Read the model definition and answer for the solid it produces. Units are mm, in the model's axes. A direction names the side the tool comes from. Give positions to 0.01 mm unless a question says otherwise; leave off trailing zeros. Order: outer loops, then holes, each group sorted by start corner. A loop starts at its lowest first (then second) coordinate and runs counter-clockwise, first axis right, second up. Notation, with made-up numbers: (-38, 31.25) - (1, 31.25) arc R23 cw to (1, 69.25) - close; hole circle Ø6 at (-9.75, 46.5). An arc over 180 degrees is marked (long way). Return JSON: item names as keys, results as strings.
```python
from build123d import *

# Parameters (mm, degrees)
F1_DEPTH  = 38.1
F2_W      = 69.85
F2_H      = 69.85
F3_DEPTH  = 127
F5_DEPTH  = 76.2
F7_DEPTH  = 25.4
F8_W      = 3.175
F8_H      = 190.3737529909
F9_DEPTH  = 3.175
F10_W     = 4.2661567543
F10_H     = 3.175
F11_DEPTH = 76.2


with BuildPart() as f1:
    # F0 (on Right) → F1 (new body, symmetric)
    with BuildSketch(Plane.YZ):
        Polygon((-76.2, 38.1), (-101.6, -38.1), (101.6, -38.1), (76.2, 38.1), align=None)
    extrude(amount=F1_DEPTH, both=True)

    # F2 (on Front) → F3 (cut, symmetric)
    with BuildSketch(Plane.XZ):
        Rectangle(F2_W, F2_H)
    extrude(amount=F3_DEPTH, both=True, mode=Mode.SUBTRACT)

    # F4 (on face) → F5 (cut)
    with BuildSketch(Plane(origin=(-38.1, 0, 0), x_dir=(0, -1, 0), z_dir=(-1, 0, 0))):
        Polygon((-71.9035431621, 34.925), (-95.1868764954, -34.925), (-71.9035431621, -34.925), align=None)
        Polygon((-66.8235431621, 27.423295483), (-66.8235431621, -34.925), (-38.1337124981, -3.7508522585), align=None)
        Polygon((-2.54, 34.925), (-66.8235431621, 34.925), (-34.6817715811, 0), align=None)
        Polygon((-2.54, -34.925), (-2.54, 27.423295483), (-31.229830664, -3.7508522585), align=None)
        Polygon((-34.6817715811, -7.501704517), (-59.9196613281, -34.925), (-9.443881834, -34.925), align=None)
        Polygon((31.229830664, -3.7508522585), (2.54, 27.423295483), (2.54, -34.925), align=None)
        Polygon((66.8235431621, 34.925), (2.54, 34.925), (34.6817715811, 0), align=None)
        Polygon((66.8235431621, -34.925), (66.8235431621, 27.423295483), (38.1337124981, -3.7508522585), align=None)
        Polygon((34.6817715811, -7.501704517), (9.443881834, -34.925), (59.9196613281, -34.925), align=None)
        Polygon((95.1868764954, -34.925), (71.9035431621, 34.925), (71.9035431621, -34.925), align=None)
    extrude(amount=-F5_DEPTH, mode=Mode.SUBTRACT)

    # F6 (on face) → F7 (cut)
    with BuildSketch(Plane.XY.offset(38.1)):
        Polygon((-34.925, 73.025), (-34.925, -58.3073754949), (-3.5194319469, 7.3588122526), align=None)
        Polygon((-34.925, -73.025), (34.925, -73.025), (0, 0), align=None)
        Polygon((3.5194319469, 7.3588122526), (34.925, -58.3073754949), (34.925, 73.025), align=None)
        Polygon((0, 14.7176245051), (27.8861361062, 73.025), (-27.8861361062, 73.025), align=None)
    extrude(amount=-F7_DEPTH, mode=Mode.SUBTRACT)

    # F8 (on face) → F9 (join)
    with BuildSketch(Plane.XY.offset(-34.925)):
        with Locations((-36.5125, 0)):
            Rectangle(F8_W, F8_H)
        with Locations((36.5125, 0)):
            Rectangle(F8_W, F8_H)
    extrude(amount=F9_DEPTH)

    # F10 (on face) → F11 (join)
    with BuildSketch(Plane.YZ.offset(38.1)):
        with Locations((-99.4669216229, -36.5125)):
            Rectangle(F10_W, F10_H)
        with Locations((99.4669216229, -36.5125)):
            Rectangle(F10_W, F10_H)
    extrude(amount=-F11_DEPTH)


solid = f1.part
```
Q1. A cutting plane is placed at A-A (x = -25). Write down the section's boundary in (y, z) (3 decimals), and give its area (3 significant figures).
Values:
{"outline": "(-101.6, -38.1) - (101.6, -38.1) - (101.6, -34.925) - (-101.6, -34.925) - close; (-77.258, 34.925) - (-73.025, 34.925) - (-73.025, 38.1) - (-76.2, 38.1) - close; (-52.273, 34.925) - (-37.555, 34.925) - (-37.555, 38.1) - (-52.273, 38.1) - close; (52.273, 34.925) - (66.99, 34.925) - (66.99, 38.1) - (52.273, 38.1) - close; (73.025, 34.925) - (77.258, 34.925) - (76.2, 38.1) - (73.025, 38.1) - close", "area": "762 mm²"}
Q2. A cutting plane is placed at B-B (y = 89). Write down the section's boundary in (x, z) (3 decimals).
Values:
{"outline": "(-38.1, -38.1) - (38.1, -38.1) - (38.1, -31.75) - (34.925, -31.75) - (34.925, -34.925) - (-34.925, -34.925) - (-34.925, -31.75) - (-38.1, -31.75) - close; (-38.1, -16.364) - (-34.925, -16.364) - (-34.925, -0.3) - (-38.1, -0.3) - close; (34.925, -16.364) - (38.1, -16.364) - (38.1, -0.3) - (34.925, -0.3) - close"}
Q3. A cutting plane is placed at D-D (z = 7.5). Give the number of separate pieces and of enclosed holes in the cut face, and give its area (3 significant figures).
Values:
{"separate pieces": "18", "enclosed holes": "0", "area": "340 mm²"}
Q4. Given pin 1 (1 mm diameter, centred on x = 37, z = -4.5, fed in from +Y); pin 2 (3.5 mm diameter, centred on x = -16.5, z = 36.5, fed in from +Y); pin 3 (1 mm diameter, centred on x = -36.5, z = 10.5, fed in from +Y), each flat-ended and moving along its own axis, determine where each tip first touches the part or whether it passes through.
Values:
{"pin 1": "stops at y = 90.57", "pin 2": "stops at y = 77.26", "pin 3": "stops at y = 85.57"}
Q5. Determine the mould class of faces 4 (the flat face through (-36.53, 82.86, 2.05)), 5 (the flat face through (34.925, -24, 9)), 6 (the flat face through (19, -25.01, 36.53)) for opening direction X: released by +X, released by -X, zero draft, split by the parting line, or undercut.
Values:
{"face 4": "zero draft", "face 5": "undercut", "face 6": "undercut"}
Q6. For faces 1 (the flat face through (-36.53, 52.28, 11.62)), 2 (the flat face through (19.44, 40.65, 36.53)), 3 (the flat face through (0.2, 76.7, 36.6)), determine the directions among +Z, -Z, +X, -X, +Y, -Y from which every point of the face is accessible in a straight line to the end or side of a thin tool.
Values:
{"face 1": "+X, -X", "face 2": "+Z", "face 3": "+Z, +X, -X, +Y"}
Q7. Consider L1, parallel to X at y = -68, z = 8 (3 decimals); L2, parallel to Z at x = -31, y = 59 (3 decimals). Determine where each line is inside the solid, lowest interval first.
Values:
{"L1": "x = -38.1 to -34.925, 34.925 to 38.1", "L2": "z = -38.1 to -34.925"}
Q8. A cutting plane is placed at C-C (y = 10). Write down the section's boundary in (x, z) (3 decimals), and give its area (3 significant figures).
Values:
{"outline": "(-38.1, -38.1) - (38.1, -38.1) - (38.1, -26.819) - (34.925, -26.819) - (34.925, -34.925) - (-34.925, -34.925) - (-34.925, -26.819) - (-38.1, -26.819) - close; (-38.1, 19.317) - (-34.925, 19.317) - (-34.925, 26.819) - (-38.1, 26.819) - close; (-38.1, 34.925) - (-34.925, 34.925) - (-34.925, 38.1) - (-38.1, 38.1) - close; (-4.783, 34.925) - (4.783, 34.925) - (4.783, 38.1) - (-4.783, 38.1) - close; (34.925, 19.317) - (38.1, 19.317) - (38.1, 26.819) - (34.925, 26.819) - close; (34.925, 34.925) - (38.1, 34.925) - (38.1, 38.1) - (34.925, 38.1) - close", "area": "392 mm²"}
